```python
from build123d import *

# Parameters (mm, degrees)
EXTRUDE1_DEPTH     = 44.45
SKETCH8_W          = 820.295635457
SKETCH8_H          = 609.826953774
CUT_EXTRUDE1_DEPTH = 38.1


with BuildPart() as part:
    # Sketch2 → Extrude1 (new body)
    with BuildSketch(Plane.XY):
        with BuildLine():
            Line((236.701314765, -109.52926958), (237.322551245, -104.518285004))
            ThreePointArc((237.322551245, -104.518285004), (238.832324595, -101.654790046), (241.859816, -100.5087906))
            Line((241.859816, -100.5087906), (287.627187, -100.5087906))
            ThreePointArc((287.627187, -100.5087906), (290.860079204, -101.847898396), (292.199187, -105.0807906))
            Line((292.199187, -105.0807906), (292.199187, -149.0184218))
            ThreePointArc((292.199187, -149.0184218), (292.597958053, -151.927621282), (293.795193618, -154.608868562))
            ThreePointArc((293.795193618, -154.608868562), (293.913773723, -154.790051229), (294.036001367, -154.968793512))
            ThreePointArc((294.036001367, -154.968793512), (296.462850079, -159.222895043), (298.58610753, -163.636368995))
            ThreePointArc((298.58610753, -163.636368995), (298.881112709, -164.165143005), (299.271135507, -164.628297651))
            ThreePointArc((299.271135507, -164.628297651), (300.007264707, -165.356749106), (300.73644663, -166.092154739))
            ThreePointArc((300.73644663, -166.092154739), (309.134939866, -171.428010927), (319.025875401, -172.512189948))
            ThreePointArc((319.025875401, -172.512189948), (322.667874381, -171.899747758), (326.235195219, -170.94399463))
            ThreePointArc((326.235195219, -170.94399463), (334.736991182, -166.788776714), (341.69241097, -160.372507853))
            ThreePointArc((341.69241097, -160.372507853), (350.978860141, -145.938116384), (356.931481894, -129.839790708))
            ThreePointArc((356.931481894, -129.839790708), (358.444492908, -124.360678247), (360.217684146, -118.960153409))
            ThreePointArc((360.217684146, -118.960153409), (361.726955491, -115.496522091), (363.691265694, -112.269119525))
            ThreePointArc((363.691265694, -112.269119525), (377.452236791, -104.634981944), (392.000789341, -110.63364853))
            ThreePointArc((392.000789341, -110.63364853), (394.334174265, -113.548333419), (396.320318679, -116.709868421))
            ThreePointArc((396.320318679, -116.709868421), (399.985801408, -125.076496738), (402.069054575, -133.970106202))
            ThreePointArc((402.069054575, -133.970106202), (402.850473596, -158.142444635), (398.510836922, -181.934882814))
            ThreePointArc((398.510836922, -181.934882814), (396.712752953, -187.660630305), (394.711731045, -193.318651304))
            ThreePointArc((394.711731045, -193.318651304), (391.254221541, -202.284530505), (387.604313736, -211.173823775))
            ThreePointArc((387.604313736, -211.173823775), (384.645418623, -218.559200445), (381.97307243, -226.053025547))
            ThreePointArc((381.97307243, -226.053025547), (379.220115758, -238.701804496), (378.745605361, -251.638002516))
            ThreePointArc((378.745605361, -251.638002516), (381.624241727, -267.094911335), (387.005590994, -281.867983379))
            ThreePointArc((387.005590994, -281.867983379), (390.741696955, -290.562895178), (394.746018404, -299.137589848))
            ThreePointArc((394.746018404, -299.137589848), (407.105387056, -324.908404556), (417.355590006, -351.588401252))
            ThreePointArc((417.355590006, -351.588401252), (421.906718125, -366.822834456), (424.846419648, -382.448418515))
            ThreePointArc((424.846419648, -382.448418515), (426.249850723, -395.79034395), (426.367663828, -409.205362144))
            ThreePointArc((426.367663828, -409.205362144), (413.851256788, -452.11341389), (383.140740026, -484.58841212))
            ThreePointArc((383.140740026, -484.58841212), (376.726903694, -488.327090669), (369.979691238, -491.423885444))
            ThreePointArc((369.979691238, -491.423885444), (361.755548517, -494.399048058), (353.346112162, -496.801025635))
            ThreePointArc((353.346112162, -496.801025635), (351.598275163, -497.203126282), (349.837333504, -497.543278577))
            ThreePointArc((349.837333504, -497.543278577), (328.927692137, -500.563756073), (307.875617353, -502.337603226))
            ThreePointArc((307.875617353, -502.337603226), (264.647049723, -503.080365686), (221.41824861, -502.351318606))
            ThreePointArc((221.41824861, -502.351318606), (221.00580821, -502.335100706), (220.593567708, -502.314415619))
            ThreePointArc((220.593567708, -502.314415619), (201.284363819, -500.712124888), (182.091052494, -498.06080619))
            ThreePointArc((182.091052494, -498.06080619), (175.416754512, -496.721648206), (168.847112314, -494.938561263))
            ThreePointArc((168.847112314, -494.938561263), (162.119330737, -492.66041844), (155.529409804, -490.009772905))
            ThreePointArc((155.529409804, -490.009772905), (153.132812394, -488.891967619), (150.797631292, -487.650961163))
            ThreePointArc((150.797631292, -487.650961163), (116.491995751, -454.558228352), (102.514776867, -408.988030339))
            ThreePointArc((102.514776867, -408.988030339), (102.647448667, -395.681700976), (104.046018753, -382.448409448))
            ThreePointArc((104.046018753, -382.448409448), (106.98510575, -366.822864688), (111.535598588, -351.588400588))
            ThreePointArc((111.535598588, -351.588400588), (121.785921274, -324.908172846), (134.146411655, -299.137609307))
            ThreePointArc((134.146411655, -299.137609307), (138.150111982, -290.562902597), (141.885599861, -281.867999389))
            ThreePointArc((141.885599861, -281.867999389), (147.267652973, -267.095112393), (150.145582523, -251.638003757))
            ThreePointArc((150.145582523, -251.638003757), (148.821670426, -233.475790137), (143.036402463, -216.208786303))
            ThreePointArc((143.036402463, -216.208786303), (140.009349985, -208.5521602), (136.805998568, -200.967602883))
            ThreePointArc((136.805998568, -200.967602883), (133.075014503, -191.465363775), (129.82521382, -181.787988837))
            ThreePointArc((129.82521382, -181.787988837), (127.242537041, -172.460798588), (125.255618654, -162.988794966))
            ThreePointArc((125.255618654, -162.988794966), (124.573431659, -146.269657735), (127.035980496, -129.718803313))
            ThreePointArc((127.035980496, -129.718803313), (131.043720455, -119.123881134), (137.44559748, -109.77881152))
            ThreePointArc((137.44559748, -109.77881152), (140.408836969, -107.058482812), (143.665986338, -104.697984023))
            ThreePointArc((143.665986338, -104.697984023), (158.033642326, -98.861944673), (173.515606109, -97.968809036))
            ThreePointArc((173.515606109, -97.968809036), (184.337065562, -99.609972723), (194.84638863, -102.668000127))
            ThreePointArc((194.84638863, -102.668000127), (208.754429598, -108.681110615), (221.847962027, -116.306758775))
            ThreePointArc((221.847962027, -116.306758775), (231.168773326, -117.069146469), (236.701314765, -109.52926958))
        make_face()
    extrude(amount=EXTRUDE1_DEPTH)

    # Sketch8 → Cut-Extrude1 (cut)
    with BuildSketch(Plane(origin=(0, 0, 0), x_dir=(-1, 0, 0), z_dir=(0, 0, -1))):
        with Locations((-256.741670113, -315.378342919)):
            Rectangle(SKETCH8_W, SKETCH8_H)
    extrude(amount=-CUT_EXTRUDE1_DEPTH, mode=Mode.SUBTRACT)


solid = part.part
```
Here's how the part is built. I have some questions about the finished solid (model axes, mm). A direction names the side the tool comes from. Round coordinates to 2 decimals unless told otherwise and drop trailing zeros. Write each loop counter-clockwise with the first axis right and the second up, starting at its lowest first coordinate (ties: lowest second). Pieces come first, ordered by that corner, then holes.
Q1. Please list where these lines run through material, in increasing order: probe 1 along Y at (x, z) = (269, 40); probe 2 along X at (y, z) = (-246, 38.75); probe 3 along X at (y, z) = (-407, 38.75).
Q2. If we section it at A-A on y = -141: Write out the boundary of the cut face in (x, z).
Q3. Will these pins go through, and if not, where does the flat tip stop? P1, Ø1.9, axis at x = 258.5, z = 41, coming from the +Y side; P2, Ø3, axis at x = 225, z = 42, coming from the +Y side; P3, Ø2, axis at y = -197, z = 43.5, coming from the -X side.
Q4. If we section it at B-B on x = 189.5: Write out the boundary of the cut face in (y, z).
Q5. If we mould it in two halves opening along X, with no side actions, what happens to faces 1 (the cylindrical face through (130.97, -119.265, 41.231)), 2 (the cylindrical face through (406.947, -324.541, 41.231)), 3 (the flat face through (267, -298, 44.45)), 4 (the cylindrical face through (350.871, -146.153, 41.231))? For each: +X half, -X half, draft (parallel to the pull), parting line (faces both ways), or undercut.
Q6. Which directions (+Z, -Z, +X, -X, +Y, -Y) give clear straight access to the entire face, cutting with the end or side of a thin tool? Please do faces 5 (the cylindrical face through (147.21, -267.31, 41.23)), 6 (the cylindrical face through (414.164, -451.564, 41.231)), 7 (the cylindrical face through (208.565, -108.586, 41.231)), 8 (the cylindrical face through (381.566, -266.882, 41.231)).
Q7. If we section it at C-C on y = -365: Write out the boundary of the cut face in (x, z), plus the area to 3 significant figures.
Answer below:
1. probe 1: y = -503.07 to -100.51
1. probe 2: x = 150.22 to 378.67
1. probe 3: x = 102.45 to 426.44
2. outline: (125.01, 38.1) - (292.2, 38.1) - (292.2, 44.45) - (125.01, 44.45) - close; (353.24, 38.1) - (402.83, 38.1) - (402.83, 44.45) - (353.24, 44.45) - close
3. P1: stops at y = -100.51
3. P2: stops at y = -117.19
3. P3: stops at x = 134.79
4. outline: (-499.21, 38.1) - (-100.92, 38.1) - (-100.92, 44.45) - (-499.21, 44.45) - close
5. face 1: -X half
5. face 2: +X half
5. face 3: draft
5. face 4: undercut
6. face 5: +Z, -Z, -X
6. face 6: +Z, -Z, +X, -Y
6. face 7: +Z, -Z, +Y
6. face 8: +Z, -Z, +X
7. outline: (107.44, 38.1) - (421.45, 38.1) - (421.45, 44.45) - (107.44, 44.45) - close
7. area: 1,990 mm2
